Input: part model. Units: mm. Frame: model coordinates. Face numbers are marked on the shaded views. Give positions to 0.01 mm unless a question says otherwise; leave off trailing zeros. Loops run counter-clockwise (first coordinate to the right, second up) from the corner with the lowest first, then second, coordinate; pieces in that order, holes last. Notation, with made-up numbers: M 46,22 L 71,22 A10 cw 71,29 Z; hole C -33,-8 d2. An arc over 180 degrees is marked long. Answer as a JSON object with one key per item and string values. Group by question number.
1) Ray query, L1, parallel to X at y = 36, z = 48.5; L2, parallel to X at y = 8.5, z = 31; L3, parallel to Y at x = -36.5, z = 23. Return the intervals inside material, ascending.
2) Draft query along X for the marked faces 1, 2 and 3. Return one class per face: +X half, -X half, draft (parallel to the pull), parting line (faces both ways), or undercut.
3) Section query B-B on x = 19. Return loops of the section in (y, z).
4) Section query C-C on z = 11. Return loops of the section in (x, y).
5) Section query D-D on y = 31.5. Return loops of the section in (x, z), plus the area to 3 significant figures.
6) Section query A-A on y = 15.5. Return loops of the section in (x, z), plus the area to 3 significant figures.
7) First-contact query: P1, Ø4, axis at x = -23, z = 9, coming from the -Y side; P2, Ø12, axis at x = 17.5, y = 44.5, coming from the +Z side; P3, Ø4, axis at x = -9, y = 28.5, coming from the +Z side. Flat tips, straight axial feed; report the tip coordinate or a pass-through.
from build123d import *

# Parameters (mm, degrees)
F0_W     = 100
F0_H     = 100
F2_DEPTH = 52
F4_DEPTH = 50
F5_R     = 50
F6_DEPTH = 100
F7_R     = 45
F8_DEPTH = 100


with BuildPart() as f2:
    # F0 (on Top) → F2 (new body)
    with BuildSketch(Plane.XY):
        Rectangle(F0_W, F0_H)
    extrude(amount=F2_DEPTH)

    # F3 (on offset) → F4 (intersect)
    with BuildSketch(Plane.YZ.offset(55.802872)):
        with BuildLine():
            ThreePointArc((25, 14.303062), (0, 28.606123), (-25, 14.303062))
            ThreePointArc((-25, 14.303062), (-39.401194, 10.474585), (-50, 0))
            ThreePointArc((-50, 0), (-25.265238, 5.467368), (0, 7.302669))
            ThreePointArc((0, 7.302669), (25.265238, 5.467368), (50, 0))
            ThreePointArc((50, 0), (39.401194, 10.474585), (25, 14.303062))
        make_face()
    extrude(amount=-F4_DEPTH, mode=Mode.INTERSECT)

    # F5 (on Top) → F6 (join)
    with BuildSketch(Plane.XY):
        with Locations((-34.342921, 36.339563)):
            Circle(F5_R)
    extrude(amount=F6_DEPTH)

    # F7 (on offset) → F8 (intersect)
    with BuildSketch(Plane.YZ.offset(55.802872)):
        with Locations((30.916278, 32.698375)):
            Circle(F7_R)
    extrude(amount=-F8_DEPTH, mode=Mode.INTERSECT)


solid = f2.part
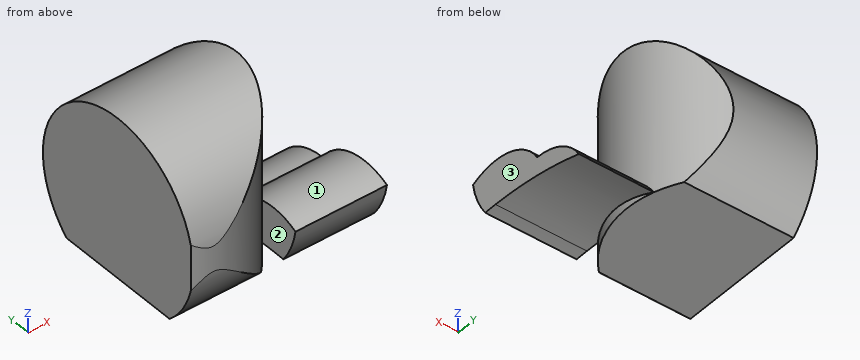
Output:
{
 "1": {"L1": "x = -44.2 to 15.66", "L2": "x = -44.2 to 7.19", "L3": "y = -13.03 to 74.86"},
 "2": {"face 1": "draft", "face 2": "undercut", "face 3": "+X half"},
 "3": {"outline": "M -13.47,25.29 A45 ccw -6.16,7.19 A174.82 cw 0,7.3 A174.82 cw 50,0 A29 ccw 25,14.3 A29 ccw Z"},
 "4": {"outline": "M -44.2,-8.51 L -12.23,-8.51 A50 ccw 5.8,6.53 L 5.8,-8.51 L 50,-8.51 L 50,38.44 L 15.61,38.44 A50 ccw 2.32,70.34 L -44.2,70.34 Z"},
 "5": {"outline": "M -44.2,0 L 15.42,0 L 15.42,4.44 L 50,4.44 L 50,13.57 L 15.42,13.57 L 15.42,77.69 L -44.2,77.69 Z", "area": "4,950 mm^2"},
 "6": {"outline": "M -44.2,0 L 11.11,0 L 11.11,6.61 L 50,6.61 L 50,24.12 L 11.11,24.12 L 11.11,74.98 L -44.2,74.98 Z", "area": "4,830 mm^2"},
 "7": {"P1": "stops at y = -8.51", "P2": "stops at z = 77", "P3": "stops at z = 77.7"}
}
